Read the model definition and answer for the solid it produces. Units are mm, in the model's axes. Face numbers are marked on the shaded views. A direction names the side the tool comes from. Round coordinates to 2 decimals unless told otherwise and drop trailing zeros. Write each loop counter-clockwise with the first axis right and the second up, starting at its lowest first coordinate (ties: lowest second). Pieces come first, ordered by that corner, then holes. Notation, with made-up numbers: (-29.75, 38.25) - (11.25, 38.25) arc R23 cw to (11.25, 47.25) - close; hole circle Ø1 at (20, 9). An arc over 180 degrees is marked (long way). Answer as CSV lines item,"result". Start each with the question number.
1) Find section C-C on y = 2.75. Determine the outline of the cut face in (x, z).
2) Find section B-B on y = 0. Determine the outline of the cut face in (x, z).
3) Consider line 1 along X through (y, z) = (3.75, 1); line 2 along Y through (x, z) = (-4.25, 0.95); line 3 along Y through (x, z) = (2, 0.5). Determine where each line is inside the solid, lowest interval first.
4) Which of the six approach directions +Z, -Z, +X, -X, +Y, -Y give full straight-line access (tool end or side, diameter ignored) to the marked faces 1 and 2?
5) Find section D-D on z = 0.8. Determine the outline of the cut face in (x, y).
6) This flat-tipped pin is pushed along its axis until it touches: pin 1 (0.6 mm diameter, centred on y = 5, z = 1, fed in from -X). Where does it stop, or does it pass through?
7) Find section A-A on x = 0. Determine the outline of the cut face in (y, z), then the cut area to 3 significant figures.
8) For a pull along X with two mould halves and no side action, classify the marked faces 3, 4 and 5 as +X half, -X half, draft (parallel to the pull), parting line (faces both ways), or undercut.
from build123d import *

# Parameters (mm, degrees)
ESQUISSE1_R             = 10
BOSS_EXTRU_1_DEPTH      = 1.3
ENL_V_MAT_EXTRU_1_DEPTH = 2.3
ESQUISSE3_R             = 1.25
ENL_V_MAT_EXTRU_2_DEPTH = 2.3


with BuildPart() as part:
    # Esquisse1 → Boss.-Extru.1 (new body)
    with BuildSketch(Plane.XY):
        Circle(ESQUISSE1_R)
    extrude(amount=BOSS_EXTRU_1_DEPTH)

    # Esquisse2 → Enlèv. mat.-Extru.1 (cut, through all)
    with BuildSketch(Plane.XY.offset(1.3)):
        with BuildLine():
            Line((-7.293475176, -3.287129425), (-2.45121915, -0.491451605))
            ThreePointArc((-2.45121915, -0.491451605), (-2.165063509, 1.25), (-0.8, 2.368543856))
            Line((-0.8, 2.368543856), (-0.8, 7.959899497))
            ThreePointArc((-0.8, 7.959899497), (-6.92820323, 4), (-7.293475176, -3.287129425))
        make_face()
        with BuildLine():
            Line((-6.493475176, -4.672770071), (-1.65121915, -1.877092251))
            ThreePointArc((-1.65121915, -1.877092251), (0, -2.5), (1.65121915, -1.877092251))
            Line((1.65121915, -1.877092251), (6.493475176, -4.672770071))
            ThreePointArc((6.493475176, -4.672770071), (0, -8), (-6.493475176, -4.672770071))
        make_face()
        with BuildLine():
            Line((2.45121915, -0.491451605), (7.293475176, -3.287129425))
            ThreePointArc((7.293475176, -3.287129425), (6.92820323, 4), (0.8, 7.959899497))
            Line((0.8, 7.959899497), (0.8, 2.368543856))
            ThreePointArc((0.8, 2.368543856), (2.165063509, 1.25), (2.45121915, -0.491451605))
        make_face()
    extrude(amount=-ENL_V_MAT_EXTRU_1_DEPTH, mode=Mode.SUBTRACT)

    # Esquisse3 → Enlèv. mat.-Extru.2 (cut, through all)
    with BuildSketch(Plane.XY.offset(1.3)):
        Circle(ESQUISSE3_R)
    extrude(amount=-ENL_V_MAT_EXTRU_2_DEPTH, mode=Mode.SUBTRACT)


solid = part.part
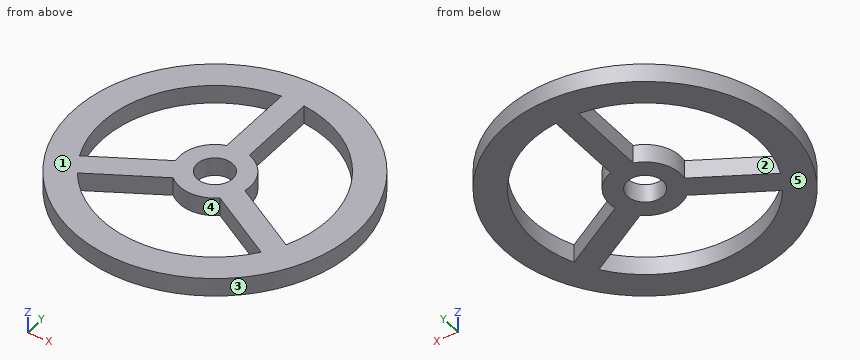
Check values:
1,outline,"(-9.61, 0) - (-7.51, 0) - (-7.51, 1.3) - (-9.61, 1.3) - close; (-0.8, 0) - (0.8, 0) - (0.8, 1.3) - (-0.8, 1.3) - close; (7.51, 0) - (9.61, 0) - (9.61, 1.3) - (7.51, 1.3) - close"
2,outline,"(-10, 0) - (-8, 0) - (-8, 1.3) - (-10, 1.3) - close; (-2.5, 0) - (-1.25, 0) - (-1.25, 1.3) - (-2.5, 1.3) - close; (1.25, 0) - (2.5, 0) - (2.5, 1.3) - (1.25, 1.3) - close; (8, 0) - (10, 0) - (10, 1.3) - (8, 1.3) - close"
3,line 1,"x = -9.27 to -7.07, -0.8 to 0.8, 7.07 to 9.27"
3,line 2,"y = -9.05 to -6.78, -3.38 to -1.53, 6.78 to 9.05"
3,line 3,"y = -9.8 to -7.75, -2.08 to 1.5, 7.75 to 9.8"
4,face 1,"+Z, +X, -X, +Y, -Y"
4,face 2,"+Z, -Z"
5,outline,"circle Ø20 at (0, 0); hole (-7.29, -3.29) - (-2.45, -0.49) arc R2.5 cw to (-0.8, 2.37) - (-0.8, 7.96) arc R8 ccw to start; hole (-6.49, -4.67) arc R8 ccw to (6.49, -4.67) - (1.65, -1.88) arc R2.5 cw to (-1.65, -1.88) - close; hole circle Ø2.5 at (0, 0); hole (0.8, 2.37) arc R2.5 cw to (2.45, -0.49) - (7.29, -3.29) arc R8 ccw to (0.8, 7.96) - close"
6,pin 1,"stops at x = -8.83"
7,outline,"(-10, 0) - (-8, 0) - (-8, 1.3) - (-10, 1.3) - close; (-2.5, 0) - (-1.25, 0) - (-1.25, 1.3) - (-2.5, 1.3) - close; (1.25, 0) - (10, 0) - (10, 1.3) - (1.25, 1.3) - close"
7,area,"15.6 mm^2"
8,face 3,"parting line"
8,face 4,"undercut"
8,face 5,"draft"
